Build history of the part. All positions in model axes, mm. Face numbers are marked on the shaded views. A direction names the side the tool comes from. Round coordinates to 2 decimals unless told otherwise and drop trailing zeros. Write each loop counter-clockwise with the first axis right and the second up, starting at its lowest first coordinate (ties: lowest second). Pieces come first, ordered by that corner, then holes. Notation, with made-up numbers: (46.25, -28) -> (86.25, -28) arc R23 ccw to (86.25, -20) -> close; hole circle Ø1 at (-28.5, 85.5). An arc over 180 degrees is marked (long way). Answer as CSV lines item,"result".
from build123d import *

# Parameters (mm, degrees)
SKETCH1_W           = 762
SKETCH1_H           = 1066.8
BOSS_EXTRUDE1_DEPTH = 228.6
FILLET1_R           = 101.6
SKETCH2_W           = 558.8
SKETCH2_H           = 25.4
CUT_EXTRUDE1_DEPTH  = 1222.578929091
CUT_EXTRUDE2_DEPTH  = 190.5


with BuildPart() as part:
    # Sketch1 → Boss-Extrude1 (new, symmetric)
    with BuildSketch(Plane.XY):
        with Locations((0, 533.4)):
            Rectangle(SKETCH1_W, SKETCH1_H)
    extrude(amount=BOSS_EXTRUDE1_DEPTH, both=True)

    # Fillet1
    fillet1_edges = [part.edges().sort_by_distance(p)[0] for p in [
        (381, 533.4, 228.6),
        (-381, 533.4, 228.6),
    ]]
    fillet(fillet1_edges, radius=FILLET1_R)

    # Sketch2 → Cut-Extrude1 (cut, through all)
    with BuildSketch(Plane.XY.offset(228.6)):
        with Locations((0, 12.7)):
            Rectangle(SKETCH2_W, SKETCH2_H)
    extrude(amount=-CUT_EXTRUDE1_DEPTH, mode=Mode.SUBTRACT)

    # Sketch3 → Cut-Extrude2 (cut, symmetric)
    with BuildSketch(Plane(origin=(0, 0, 0), x_dir=(0, 0, -1), z_dir=(1, 0, 0))):
        Polygon((-152.4, 1066.8), (-228.6, 782.417728463), (-228.6, 1066.8), align=None)
    extrude(amount=CUT_EXTRUDE2_DEPTH, both=True, mode=Mode.SUBTRACT)


solid = part.part
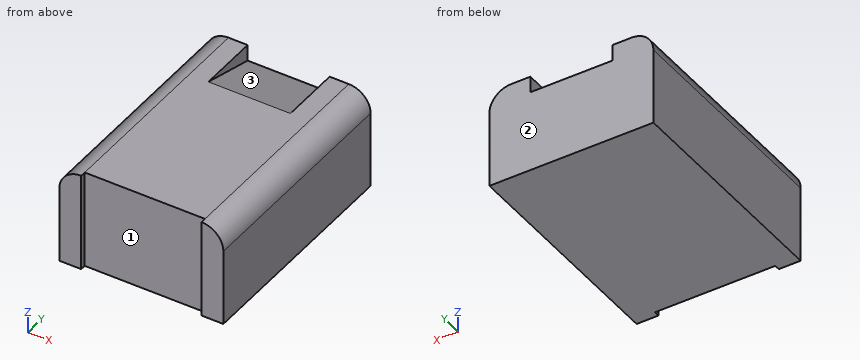
1. Probe line 1 along Y through (x, z) = (101, -64); line 2 along X through (y, z) = (107.5, 134); line 3 along Z through (x, y) = (280, 665.5). List the from-to ranges inside material, lowest first.
Results found:
line 1,"y = 25.4 to 1066.8"
line 2,"x = -380.76 to 380.76"
line 3,"z = -228.6 to 228.6"
2. Which spindle directions (+Z, -Z, +X, -X, +Y, -Y) get a long thin tool onto all of the face, cutting with end or side? Do the marked faces 1, 2 and 3. Say none if no direction does.
Results found:
face 1,"+Z, -Z, -Y"
face 2,"+Z, -Z, +X, -X, +Y"
face 3,"+Z, +Y"
3. Cut at D-D, the plane x = 247.5. Write the cut outline in (y, z), then the cut area to 3 significant figures.
Results found:
outline,"(25.4, -228.6) -> (1066.8, -228.6) -> (1066.8, 228.6) -> (25.4, 228.6) -> close"
area,"476,000 mm2"
4. Cut at B-B, the plane x = -147.5. Write the cut outline in (y, z).
Results found:
outline,"(25.4, -228.6) -> (1066.8, -228.6) -> (1066.8, 152.4) -> (782.42, 228.6) -> (25.4, 228.6) -> close"
5. Drop flat-ended pins along their axis: pin 1 Ø8 at (x, z) = (-116, 171.5) entering from -Y; pin 2 Ø10 at (y, z) = (675, 181.5) entering from +X; pin 3 Ø23 at (y, z) = (956, 172) entering from +X. Give the stop position or say it passes through.
Results found:
pin 1,"stops at y = 25.4"
pin 2,"stops at x = 368.13"
pin 3,"stops at x = 375.32"
6. Cut at A-A, the plane z = -134. Write the cut outline in (x, y).
Results found:
outline,"(-381, 0) -> (-279.4, 0) -> (-279.4, 25.4) -> (279.4, 25.4) -> (279.4, 0) -> (381, 0) -> (381, 1066.8) -> (-381, 1066.8) -> close"
7. Cut at C-C, the plane y = 829. Write the cut outline in (x, z).
Results found:
outline,"(-381, -228.6) -> (381, -228.6) -> (381, 127) arc R101.6 ccw to (279.4, 228.6) -> (190.5, 228.6) -> (190.5, 216.12) -> (-190.5, 216.12) -> (-190.5, 228.6) -> (-279.4, 228.6) arc R101.6 ccw to (-381, 127) -> close"
